The figure shows three views and two pictorial views of one solid part (mm, origin at its lowest corner). Answer the questions. A direction names the side the tool comes from. Coordinates: 2 decimals unless noted, no trailing zeros. Loops run counter-clockwise (first coordinate to the right, second up) from the corner with the lowest first, then second, coordinate; pieces in that order, holes last. Notation, with made-up numbers: (-1, 39) -> (26, 39) arc R26 ccw to (26, 65) -> close; hole circle Ø6 at (60.5, -21.5). An arc over 180 degrees is marked (long way). Answer as a JSON object with one key per item and string values. Group by question number.
1) Section D-D, the plane y = 5.45 is taken. Give the vertices of the cut face in (x, z).
2) Section C-C, the plane z = 8.5 is taken. Give the vertices of the cut face in (x, y).
3) Which of the six approach directions +Z, -Z, +X, -X, +Y, -Y give full straight-line access (tool end or side, diameter ignored) to the marked faces 1, 2 and 3?
4) Flat-ended cylindrical pins translate along their axes: P1, Ø1.5, axis at x = 2, z = 12, coming from the -Y side; P2, Ø0.7, axis at y = 1.5, z = 5.5, coming from the +X side; P3, Ø2, axis at y = 4.5, z = 10, coming from the +X side. Find the tip coordinate at first contact, or state that the pin passes through.
5) Section A-A, the plane x = 3 is taken. Give the vertices of the cut face in (y, z), plus the area to 3 significant figures.
6) Consider probe 1 along X at (y, z) = (1.8, 12.5); probe 2 along X at (y, z) = (2.9, 4.5). Determine where each line is inside the solid, lowest interval first. Write a range as [from, to].
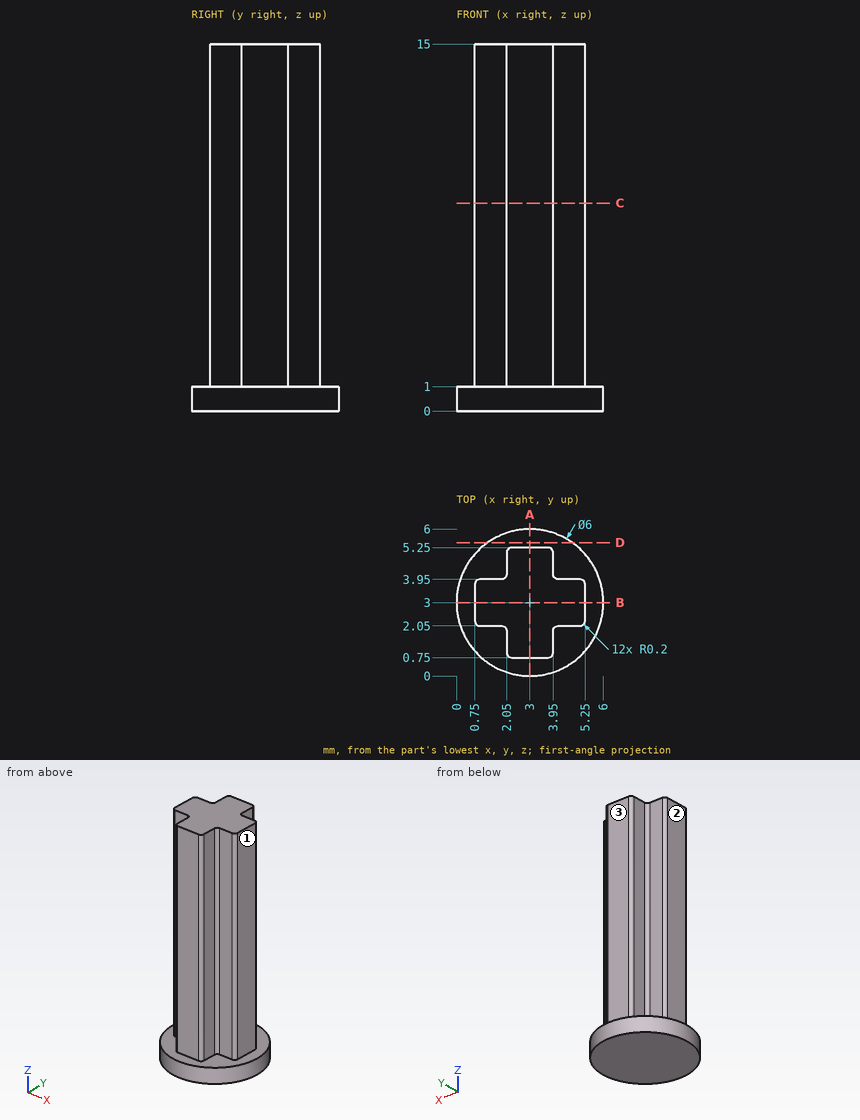
Determined:
{
 "1": {"outline": "(1.27, 0) -> (4.73, 0) -> (4.73, 1) -> (1.27, 1) -> close"},
 "2": {"outline": "(0.75, 2.25) arc R0.2 ccw to (0.95, 2.05) -> (1.85, 2.05) arc R0.2 cw to (2.05, 1.85) -> (2.05, 0.95) arc R0.2 ccw to (2.25, 0.75) -> (3.75, 0.75) arc R0.2 ccw to (3.95, 0.95) -> (3.95, 1.85) arc R0.2 cw to (4.15, 2.05) -> (5.05, 2.05) arc R0.2 ccw to (5.25, 2.25) -> (5.25, 3.75) arc R0.2 ccw to (5.05, 3.95) -> (4.15, 3.95) arc R0.2 cw to (3.95, 4.15) -> (3.95, 5.05) arc R0.2 ccw to (3.75, 5.25) -> (2.25, 5.25) arc R0.2 ccw to (2.05, 5.05) -> (2.05, 4.15) arc R0.2 cw to (1.85, 3.95) -> (0.95, 3.95) arc R0.2 ccw to (0.75, 3.75) -> close"},
 "3": {"face 1": "+Z, +X, +Y, -Y", "face 2": "+Z, -X, +Y, -Y", "face 3": "+Z, +X, -X, +Y"},
 "4": {"P1": "y = 0.75", "P2": "x = 3.95", "P3": "x = 5.25"},
 "5": {"outline": "(0, 0) -> (6, 0) -> (6, 1) -> (5.25, 1) -> (5.25, 15) -> (0.75, 15) -> (0.75, 1) -> (0, 1) -> close", "area": "69.0 mm²"},
 "6": {"probe 1": "[2.05, 3.95]", "probe 2": "[0.75, 5.25]"}
}
